The model under review builds one solid part; all positions refer to its coordinate system, in mm. A direction names the side the tool comes from. Round coordinates to 2 decimals unless told otherwise and drop trailing zeros. Write each loop counter-clockwise with the first axis right and the second up, starting at its lowest first coordinate (ties: lowest second). Pieces come first, ordered by that corner, then holes. Notation, with made-up numbers: (32.5, -33.75) - (81.5, -33.75) arc R33 cw to (81.5, 3.25) - close; hole circle Ø5 at (44, 25). An arc over 180 degrees is marked (long way). Return JSON: item names as keys, results as strings.
from build123d import *

# Parameters (mm, degrees)
BOSS_EXTRUDE1_DEPTH = 3


with BuildPart() as part:
    # Sketch1 → Boss-Extrude1 (new body)
    with BuildSketch(Plane(origin=(0, 0, 0), x_dir=(1, 0, 0), z_dir=(0, 1, 0))):
        with BuildLine():
            Line((0, 0), (61.5, 0))
            add(Edge.make_bspline(
                [(61.5, 0), (96.079868576, 1.689945504), (120.026085552, 10.3)],
                knots=[0, 0, 0, 1, 1, 1], degree=2))
            Line((120.026085552, 10.3), (120.028762053, 16.803234674))
            add(Edge.make_bspline(
                [(61.5, 6.5), (96.082545077, 8.193180177), (120.028762053, 16.803234674)],
                knots=[0, 0, 0, 1, 1, 1], degree=2))
            Line((61.5, 6.5), (0, 6.5))
            Line((0, 6.5), (-3, 6.5))
            Line((-3, 6.5), (-3, 0))
            Line((-3, 0), (0, 0))
        make_face()
    extrude(amount=BOSS_EXTRUDE1_DEPTH)


solid = part.part
(1) Add section A-A (x = 45). Write out the cut boundary in (y, z), plus the area to 3 significant figures.
Filled in:
{"outline": "(0, -6.5) - (3, -6.5) - (3, 0) - (0, 0) - close", "area": "19.5 mm2"}
(2) Clearance check with flat-ended pins moving along their axes: pin 1 Ø1.5 at (x, y) = (78.5, 2) entering from -Z; pin 2 Ø1.5 at (x, y) = (41, 1.5) entering from -Z. State where each tip first meets the part, or that it passes through.
Filled in:
{"pin 1": "stops at z = -7.9", "pin 2": "stops at z = -6.5"}
(3) Wall thickness on line 1 (Z direction, x = 47, y = 1.9); line 2 (Z direction, x = 115, y = 0.3): over which ranges is each line inside the solid? List them lowest first.
Filled in:
{"line 1": "z = -6.5 to 0", "line 2": "z = -15.11 to -8.61"}
(4) For faces 1 (the flat face through (30, 1, -6.5)), 2 (the flat face through (58, 3, -5)), list the 3-axis set-ups (+Z, -Z, +X, -X, +Y, -Y) from which the entire face can be reached by the end or side of a thin tool; tool diameter is ignored.
Filled in:
{"face 1": "-Z, -X, +Y, -Y", "face 2": "+Z, -Z, +X, -X, +Y"}
